from build123d import *

# Parameters (mm, degrees)
F0_W     = 16
F0_H     = 16
F0_W_2   = 10
F0_H_2   = 10
F1_DEPTH = 16
F2_W     = 10
F2_H     = 10
F3_DEPTH = 25
F4_W     = 10
F4_H     = 10
F5_DEPTH = 25


with BuildPart() as f1:
    # F0 (on Top) → F1 (new body)
    with BuildSketch(Plane.XY):
        with Locations((8, 8)):
            Rectangle(F0_W, F0_H)
        with Locations((8, 8)):
            Rectangle(F0_W_2, F0_H_2, mode=Mode.SUBTRACT)
    extrude(amount=F1_DEPTH)

    # F2 (on face) → F3 (cut)
    with BuildSketch(Plane.XZ):
        with Locations((8, 8)):
            Rectangle(F2_W, F2_H)
    extrude(amount=-F3_DEPTH, mode=Mode.SUBTRACT)

    # F4 (on face) → F5 (cut)
    with BuildSketch(Plane.YZ.offset(16)):
        with Locations((8, 8)):
            Rectangle(F4_W, F4_H)
    extrude(amount=-F5_DEPTH, mode=Mode.SUBTRACT)


solid = f1.part
Source: CAD feature listing. Evaluate the final solid. Frame: model axes, mm. A direction names the side the tool comes from. Coordinates: 2 decimals unless noted, no trailing zeros. Order: outer loops, then holes, each group sorted by start corner. A loop starts at its lowest first (then second) coordinate and runs counter-clockwise, first axis right, second up.
Item 1: Set-up query: faces 4 (the face through (8, 3, 14)), 5 (the face through (13.2, 8.1, 0)), 6 (the face through (3, 14, 8)), 7 (the face through (2, 8, 3)). Return all of +Z, -Z, +X, -X, +Y, -Y with unobstructed straight access to the full face (end or side cutting, diameter ignored); none if empty.
Output values:
face 4: +Z, -Z
face 5: -Z, +X, -X, +Y, -Y
face 6: +Y, -Y
face 7: +X, -X
Item 2: First-contact query: P1, Ø1, axis at y = 11.5, z = 11, coming from the -X side. Flat tip, straight axial feed; report the tip coordinate or a pass-through.
Output values:
P1: passes through
Item 3: Pull-direction query (Y, two-part tool) for faces 1 (the face through (15, 8, 3)), 2 (the face through (15, 13, 8)), 3 (the face through (8, 14, 3)); classes: pulls with the +Y half, pulls with the -Y half, needs draft (parallel to the pull), parting line crosses it, or undercut.
Output values:
face 1: undercut
face 2: undercut
face 3: needs draft
Item 4: Material intervals for line 1 (Y direction, x = 6, z = 2.5), sorted ascending.
Output values:
line 1: y = 0 to 3, 13 to 16
Item 5: Cut plane C-C (x = 1.5). Return loops of the section in (y, z).
Output values:
outline: (0, 0) - (16, 0) - (16, 16) - (0, 16) - close; hole (3, 3) - (13, 3) - (13, 13) - (3, 13) - close
Item 6: Cut plane A-A (z = 6). Return loops of the section in (x, y).
Output values:
outline: (0, 0) - (3, 0) - (3, 3) - (0, 3) - close; (0, 13) - (3, 13) - (3, 16) - (0, 16) - close; (13, 0) - (16, 0) - (16, 3) - (13, 3) - close; (13, 13) - (16, 13) - (16, 16) - (13, 16) - close
